Study the drawing (mm; zero at the part's minimum x, y, z) and answer. A direction names the side the tool comes from. Round coordinates to 2 decimals unless told otherwise and drop trailing zeros. Write each loop counter-clockwise with the first axis right and the second up, starting at its lowest first coordinate (ties: lowest second). Pieces come first, ordered by that corner, then holes. Notation, with made-up numbers: (28.25, 3.25) -> (66.25, 3.25) arc R30 cw to (66.25, 30.25) -> close; hole circle Ø2 at (-9, -7.75). An arc over 180 degrees is marked (long way). Return JSON: item names as keys, results as strings.
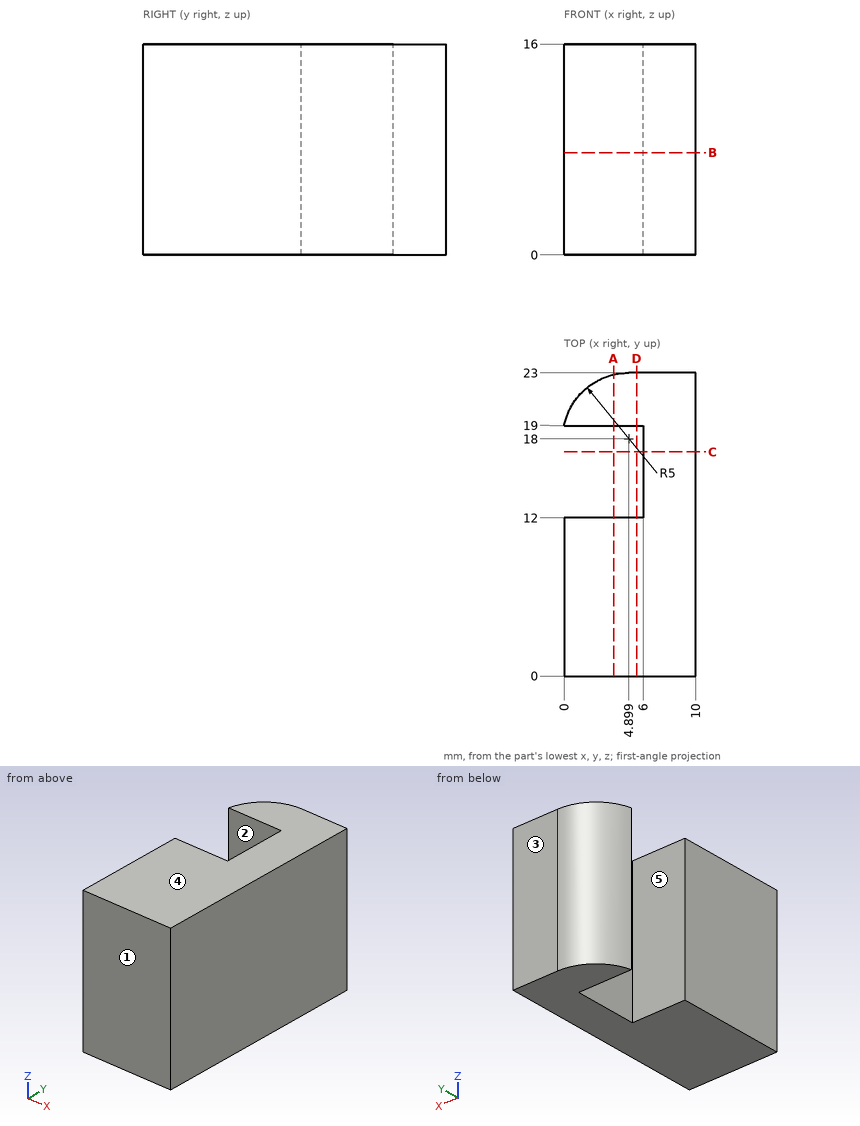
Item 1: Section C-C (y = 17) is taken. Give the vertices of the cut face in (x, z), then the cut area to 3 significant figures.
Worked answers:
{"outline": "(6, 0) -> (10, 0) -> (10, 16) -> (6, 16) -> close", "area": "64.0 mm2"}
Item 2: For a pull along Y with two mould halves and no side action, classify the marked faces 3, 4 and 5 as released by +Y, released by -Y, zero draft, split by the parting line, or undercut.
Worked answers:
{"face 3": "released by +Y", "face 4": "zero draft", "face 5": "undercut"}
Item 3: Section B-B (z = 7.75) is taken. Give the vertices of the cut face in (x, y), then the cut area to 3 significant figures.
Worked answers:
{"outline": "(0, 0) -> (10, 0) -> (10, 23) -> (4.9, 23) arc R5 ccw to (0, 19) -> (6, 19) -> (6, 12) -> (0, 12) -> close", "area": "183 mm2"}
Item 4: Straight lines are drawn through the part: L1, parallel to Y at x = 4.75, z = 9; L2, parallel to Y at x = 1.75, z = 12; L3, parallel to X at y = 17.75, z = 14. For each, find the intervals that lie inside material, in ascending order. Write a range as [from, to].
Worked answers:
{"L1": "y = [0, 12], [19, 23]", "L2": "y = [0, 12], [19, 21.88]", "L3": "x = [6, 10]"}
Item 5: Flat-ended cylindrical pins translate along their axes: pin 1 (1.5 mm diameter, centred on y = 15.5, z = 12, fed in from -X); pin 2 (1.5 mm diameter, centred on x = 3.5, y = 15, fed in from -Z). Find the tip coordinate at first contact, or state that the pin passes through.
Worked answers:
{"pin 1": "stops at x = 6", "pin 2": "passes through"}
Item 6: Section D-D (x = 5.5) is taken. Give the vertices of the cut face in (y, z).
Worked answers:
{"outline": "(0, 0) -> (12, 0) -> (12, 16) -> (0, 16) -> close; (19, 0) -> (23, 0) -> (23, 16) -> (19, 16) -> close"}
Item 7: A tool of negligible diameter and unlimited length cuts with its end or side. For the marked faces 1 and 2, from which of +Z, -Z, +X, -X, +Y, -Y can it reach the whole face along a straight path? Write none if from no direction.
Worked answers:
{"face 1": "+Z, -Z, +X, -X, -Y", "face 2": "+Z, -Z, -X"}
Item 8: Section A-A (x = 3.75) is taken. Give the vertices of the cut face in (y, z).
Worked answers:
{"outline": "(0, 0) -> (12, 0) -> (12, 16) -> (0, 16) -> close; (19, 0) -> (22.87, 0) -> (22.87, 16) -> (19, 16) -> close"}
